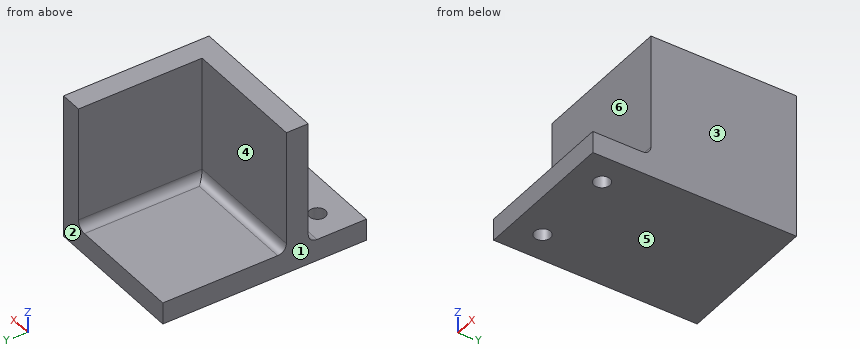
Autodesk Fusion 360 part; units mm, degrees
sketch "Sketch1" plane through (0, 0, 0) normal (0, 0, 1) x (1, 0, 0)
  line L0 (0, 0) -> (50, 0)
  line L1 (50, 0) -> (50, 50)
  line L2 (0, 7.5) -> (42.5, 7.5)
  line L3 (42.5, 7.5) -> (42.5, 50)
  line L4 (0, 7.5) -> (0, 0)
  line L5 (42.5, 50) -> (50, 50)
  dimension "d1" = -7.5
  dimension "d2" = 50
  dimension "d3" = 50
extrude "Extrude1" add sketch "Sketch1" along normal blind 50
sketch "Sketch4" plane through (0, 0, 0) normal (0, 0, 1) x (1, 0, 0)
  line L0 (50, -20) -> (0, -20)
  line L1 (0, -20) -> (0, 50)
  line L2 (0, 50) -> (50, 50)
  line L3 (50, 50) -> (50, -20)
  point P0 (50, 50)
  dimension "d43" = 70
  dimension "d44" = 50
extrude "Extrude4" add sketch "Sketch4" along normal blind 7.5
sketch "Sketch7" plane through (0, 0, 7.5) normal (0, 0, 1) x (-1, 0, 0)
  line L0 (0, 0) -> (0, 20)
  line L1 (-50, 0) -> (0, 0)
  line L2 (0, 20) -> (-50, 20)
  line L3 (-50, 20) -> (-50, 0)
  point P0 (-10, 10)
  point P1 (-40, 10)
  dimension "d35" = 30
hole "Hole1" at (10, -10, 7.5) at (40, -10, 7.5) direction (0, 0, -1) diameter 5.5 depth 10 tip angle 118
fillet "Fillet1" radius 3 1 edges at (25, 0, 7.5)
fillet "Fillet1" radius 3 2 edges at (21.25, 7.5, 7.5) (42.5, 28.75, 7.5)
Model file for the job. Use its own axes, mm. Face numbers are marked on the shaded views. A direction names the side the tool comes from. Coordinates: 2 decimals unless noted, no trailing zeros. Loops run counter-clockwise (first coordinate to the right, second up) from the corner with the lowest first, then second, coordinate; pieces in that order, holes last. Notation, with made-up numbers: (53, 55.5) - (90, 55.5) arc R25 cw to (90, 85.5) - close; hole circle Ø8 at (-16, -35). An arc over 180 degrees is marked (long way). Write item = value, one per line. Start each with the question number.
Item 1: Saw through at D-D, the plane x = 44. List the corners of the cut face in (y, z), then the cut area to 3 significant figures.
Item 2: Pull direction X, two halves, no side cores. Call the marked faces 1, 2 and 3: +X half, -X half, draft (parallel to the pull), parting line (faces both ways), or undercut.
Item 3: Drop flat-ended pins along their axis: pin 1 Ø3 at (x, z) = (30.5, 15.5) entering from +Y; pin 2 Ø5 at (x, y) = (40, -10) entering from -Z; pin 3 Ø3 at (y, z) = (16.5, 14) entering from -X; pin 4 Ø9 at (x, y) = (10, -10) entering from +Z. Give the stop position or say it passes through.
Item 4: Saw through at C-C, the plane y = 12.5. List the corners of the cut face in (x, z), then the cut area to 3 significant figures.
Item 5: Saw through at B-B, the plane x = 10. List the corners of the cut face in (y, z).
Item 6: Wall check: probe 1 along X at (y, z) = (-10, 4); probe 2 along Y at (x, z) = (40, 5); probe 3 along Z at (x, y) = (35, -6). Give the ranges that are in metal, low to high. Write a range as [from, to].
Item 7: Saw through at A-A, the plane y = -10. List the corners of the cut face in (x, z), then the cut area to 4 significant figures.
Item 8: 3-axis set-ups, long thin cutter, end or side, ignore diameter. For the marked faces 4, 5 and 6: which of +Z, -Z, +X, -X, +Y, -Y reach the whole face in a straight line?
Answers:
q1.outline = (-20, 0) - (50, 0) - (50, 50) - (0, 50) - (0, 10.5) arc R3 cw to (-3, 7.5) - (-20, 7.5) - close
q1.area = 2,650 mm2
q2.face_1 = -X half
q2.face_2 = draft
q2.face_3 = +X half
q3.pin_1 = 7.5
q3.pin_2 = through
q3.pin_3 = 42.5
q3.pin_4 = 7.5
q4.outline = (0, 0) - (50, 0) - (50, 50) - (42.5, 50) - (42.5, 10.5) arc R3 cw to (39.5, 7.5) - (0, 7.5) - close
q4.area = 696 mm2
q5.outline = (-20, 0) - (-12.75, 0) - (-12.75, 7.5) - (-20, 7.5) - close; (-7.25, 0) - (50, 0) - (50, 7.5) - (10.5, 7.5) arc R3 cw to (7.5, 10.5) - (7.5, 50) - (0, 50) - (0, 10.5) arc R3 cw to (-3, 7.5) - (-7.25, 7.5) - close
q6.probe_1 = [0, 7.25], [12.75, 37.25], [42.75, 50]
q6.probe_2 = [-20, -12.75], [-7.25, 50]
q6.probe_3 = [0, 7.5]
q7.outline = (0, 0) - (7.25, 0) - (7.25, 7.5) - (0, 7.5) - close; (12.75, 0) - (37.25, 0) - (37.25, 7.5) - (12.75, 7.5) - close; (42.75, 0) - (50, 0) - (50, 7.5) - (42.75, 7.5) - close
q7.area = 292.5 mm2
q8.face_4 = +Z, -X, +Y
q8.face_5 = -Z, +X, -X, +Y, -Y
q8.face_6 = +Z, +X, -X, -Y
